Autodesk Inventor part; units mm, degrees
ref_plane "YZ Plane" through (0, 0, 0) normal (1, 0, 0) x (0, 1, 0)
ref_plane "XZ Plane" through (0, 0, 0) normal (0, 1, 0) x (-1, 0, 0)
ref_plane "XY Plane" through (0, 0, 0) normal (0, 0, 1) x (1, 0, 0)
sketch "Sketch1" plane through (0, 0, 0) normal (0, 1, 0) x (-1, 0, 0)
  line L0 (10, -45) -> (-10, -45)
  line L1 (-10, -45) -> (-10, 47.1)
  line L2 (-10, 47.1) -> (10, 47.1)
  line L3 (10, 47.1) -> (10, -45)
  point P0 (0, 0)
  dimension "d0" = 20
  dimension "d1" = 92.1
  dimension "d2" = 45
  dimension "d3" = 10
extrude "Plate1" add sketch "Sketch1" along normal blind 1.5
sketch "Sketch2" plane through (0, 0, 0) normal (0, -1, 0) x (1, 0, 0)
  circle A0 centre (0, 42) radius 0.7835
  circle A1 centre (-7, 35) radius 0.7835
  circle A2 centre (0, 28) radius 0.7835
  circle A3 centre (7, 35) radius 0.7835
  circle A4 centre (0, -28) radius 0.7835
  circle A5 centre (-7, -35) radius 0.7835
  circle A6 centre (0, -42) radius 0.7835
  circle A7 centre (7, -35) radius 0.7835
  circle A8 centre (7, 37.1) radius 0.7835
  circle A9 centre (0, 30.1) radius 0.7835
  circle A10 centre (-7, 37.1) radius 0.7835
  circle A11 centre (0, 44.1) radius 0.7835
  point P0 (0, 0)
hole "Hole1" at (0, 0, 30.1) at (7, 0, 37.1) at (0, 0, 44.1) at (-7, 0, 37.1) at (0, 0, -42) at (7, 0, -35) at (0, 0, -28) at (-7, 0, -35) direction (0, 1, 0) diameter 2.1 depth 1.5
sketch "Sketch3" plane through (0, 1.5, 0) normal (0, 1, 0) x (1, 0, 0)
  arc A0 (10, 35) -> (-10, 35) centre (0, 35) ccw
  arc A1 (-10, -37.1) -> (10, -37.1) centre (0, -37.1) ccw
  line L0 (-10, 35) -> (-10, -37.1)
  line L1 (10, 35) -> (10, -37.1)
  line L2 (10, 45) -> (10, -47.1)
  line L3 (-10, 45) -> (10, 45)
  line L4 (10, 45) -> (10, -47.1)
  line L5 (10, -47.1) -> (-10, -47.1)
  line L6 (-10, -47.1) -> (-10, 45)
  point P0 (0, 0)
  point P1 (0, 45)
  point P2 (10, 45)
  point P3 (10, 35)
  point P4 (-10, -37.1)
  point P5 (0, -47.1)
  point P6 (1.4107, 44.9)
  point P7 (10, 35)
  dimension "d12" = 35
  dimension "d13" = 37.1
  dimension "d14" = 10
  dimension "d15" = 10
  dimension "d16" = 10
  dimension "d17" = 20
  dimension "d18" = 92.1
extrude "Extrusion1" cut sketch "Sketch3" against normal blind 10 contours A0 L3 L2 | A0 L6 L3 | L2 L5 A1 | L5 L6 A1
sketch "Sketch4" plane through (0, 1.5, 0) normal (0, 1, 0) x (1, 0, 0)
  arc A0 (10, 35) -> (-10, 35) centre (0, 35) ccw
  arc A1 (-10, -37.1) -> (10, -37.1) centre (0, -37.1) ccw
  point P0 (0, 0)
hole "Hole2" at (0, 1.5, -35) at (0, 1.5, 37.1) direction (0, -1, 0) diameter 5.2 depth 1.5
equation "\"d10\" = Thickness"
equation "\"d26\" = Thickness"
equation "\"d4\" = Thickness"
equation "\"BendReliefWidth\" = Thickness"
equation "\"BendReliefDepth\" = 0.5 * Thickness"
equation "\"CornerReliefSize\" = 4 * Thickness"
equation "\"MinimumRemnant\" = 2 * Thickness"
equation "\"TransitionRadius\" = BendRadius"
equation "\"JacobiRadiusSize\" = BendRadius"
equation "\"GapSize\" = Thickness"
properties part number "axis_10_11-connector_frame" material "Aluminum 6061-AHC"
Geometry: final body of the model. Coordinates: model frame, mm. Round coordinates to 2 decimals unless told otherwise and drop trailing zeros. Loops run counter-clockwise (first coordinate to the right, second up) from the corner with the lowest first, then second, coordinate; pieces in that order, holes last.
Q1. Section D-D on x = -7. Return loops of the section in (y, z), plus the area to 3 significant figures.
Q2. Material intervals for L1, parallel to X at y = 0.8, z = 37; L2, parallel to Z at x = 7.5, y = 1.1; L3, parallel to X at y = 1.15, z = 30.1, sorted ascending.
Q3. Section C-C on y = 0.45. State how many separate pieces and enclosed holes the cut face has, plus the area to 3 significant figures.
Q4. Section B-B on z = 30.1. Return loops of the section in (x, y), plus the area to 4 significant figures.
Q5. Pull-direction query (X, two-part tool) for faces 1 (the cylindrical face through (0, 1, -45)), 2 (the flat face through (-10, 1, 2)), 3 (the cylindrical face through (-0.32, 0.76, 43.1)), 4 (the cylindrical face through (0.4, 0.76, -28.97)); classes: released by +X, released by -X, zero draft, split by the parting line, or undercut.
Q6. Section A-A on x = 0. Return loops of the section in (y, z), plus the area to 3 significant figures.
Evaluation:
1. outline: (0, -42.14) - (1.5, -42.14) - (1.5, -36.05) - (0, -36.05) - close; (0, -33.95) - (1.5, -33.95) - (1.5, 36.05) - (0, 36.05) - close; (0, 38.15) - (1.5, 38.15) - (1.5, 44.24) - (0, 44.24) - close
1. area: 123 mm2
2. L1: x = -10 to -8.05, -5.95 to -2.6, 2.6 to 5.95, 8.05 to 10
2. L2: z = -41.61 to -35.92, -34.08 to 36.18, 38.02 to 43.71
2. L3: x = -10 to -1.05, 1.05 to 10
3. separate pieces: 1
3. enclosed holes: 10
3. area: 1,690 mm2
4. outline: (-10, 0) - (-1.05, 0) - (-1.05, 1.5) - (-10, 1.5) - close; (1.05, 0) - (10, 0) - (10, 1.5) - (1.05, 1.5) - close
4. area: 26.85 mm2
5. face 1: split by the parting line
5. face 2: released by -X
5. face 3: undercut
5. face 4: undercut
6. outline: (0, -45) - (1.5, -45) - (1.5, -43.05) - (0, -43.05) - close; (0, -40.95) - (1.5, -40.95) - (1.5, -37.6) - (0, -37.6) - close; (0, -32.4) - (1.5, -32.4) - (1.5, -29.05) - (0, -29.05) - close; (0, -26.95) - (1.5, -26.95) - (1.5, 29.05) - (0, 29.05) - close; (0, 31.15) - (1.5, 31.15) - (1.5, 34.5) - (0, 34.5) - close; (0, 39.7) - (1.5, 39.7) - (1.5, 43.05) - (0, 43.05) - close; (0, 45.15) - (1.5, 45.15) - (1.5, 47.1) - (0, 47.1) - close
6. area: 110 mm2
